Could you check a few things on this model? Use its own coordinates, in mm. A direction names the side the tool comes from. Give positions to 0.01 mm unless a question says otherwise; leave off trailing zeros. Write each loop counter-clockwise with the first axis right and the second up, starting at its lowest first coordinate (ties: lowest second). Pieces come first, ordered by that corner, then holes. Notation, with made-up numbers: (40, 9) - (96, 9) arc R27 ccw to (96, 35) - close; hole circle Ø6 at (75, 41). An arc over 180 degrees is marked (long way). Use one line per item in the form item = value.
Autodesk Inventor part; units mm, degrees
ref_plane "YZ Plane" through (0, 0, 0) normal (1, 0, 0) x (0, 1, 0)
ref_plane "XZ Plane" through (0, 0, 0) normal (0, 1, 0) x (-1, 0, 0)
ref_plane "XY Plane" through (0, 0, 0) normal (0, 0, 1) x (1, 0, 0)
sketch "Sketch1" plane through (0, 0, 0) normal (0, 1, 0) x (-1, 0, 0)
  line L0 (0, 0) -> (22.5, 0)
  line L1 (22.5, 0) -> (22.5, -21)
  line L2 (22.5, -21) -> (0, -21)
  line L3 (0, -21) -> (0, 0)
  circle A0 centre (3, -3) radius 1.5
  circle A1 centre (3, -18) radius 1.5
  line L4 (22.5, -10.5) -> (0, -10.5)
  dimension "d0" = 21
  dimension "d1" = 22.5
  dimension "d2" = 3
  dimension "d5" = 3
  dimension "d8" = 3
  dimension "d25" = 15
  dimension "d26" = 3
extrude "Extrusion1" add sketch "Sketch1" along normal blind 1.5
sketch "Sketch2" plane through (0, 1.5, 0) normal (0, 1, 0) x (1, 0, 0)
  line L0 (-3, 7) -> (-1, 7)
  line L1 (-1, 7) -> (-1, 14)
  line L2 (-1, 14) -> (-3, 14)
  line L3 (-3, 14) -> (-3, 7)
  line L4 (-16.5, 8.25) -> (-16.5, 12.75)
  circle A0 centre (-16.5, 10.5) radius 2.25
  line L5 (-22.5, 21) -> (-22.5, 0)
  line L6 (-22.5, 10.5) -> (0, 10.5)
  line L7 (0, 0) -> (0, 21)
  dimension "d11" = 4.5
  dimension "d12" = 7
  dimension "d13" = 2
  dimension "d14" = 1
  dimension "d15" = 6
extrude "Extrusion2" add sketch "Sketch2" along normal blind 4.5 contours L3 L6 L1 L0 | A0 L4 L6 | L6 L4 A0 | L3 L2 L1 L6 picked at (-15.2379, 9.707) picked at (-15.707, 11.7621)
sketch "Sketch3" plane through (-1, 1.5, -7) normal (1, 0, 0) x (0, 0, -1)
  line L0 (0.5, 3.5) -> (6.5, 3.5)
  line L1 (6.5, 3.5) -> (6.5, 4.5)
  line L2 (6.5, 4.5) -> (0.5, 4.5)
  line L3 (0.5, 4.5) -> (0.5, 3.5)
  line L4 (-7, 0) -> (14, 0)
  line L5 (0, 4.5) -> (7, 4.5)
  line L6 (0, 0) -> (0, 4.5)
  line L7 (7, 0) -> (7, 4.5)
  point P0 (-7, -1.5)
  point P1 (0.5, 4)
  dimension "d18" = 6
  dimension "d19" = 1
  dimension "d21" = 0.5
  dimension "d22" = 0.5
extrude "Extrusion3" add sketch "Sketch3" along normal blind 8 contours L3 L2 L1 L0
properties part number "DS18B20"
1. Imagine slicing it at B-B, the plane y = 4.2. List the corners of the cut face in (x, z) for me.
Response values:
outline = (-16.5, -12.75) arc R2.25 ccw to (-16.5, -8.25) - close; (-3, -14) - (-1, -14) - (-1, -7) - (-3, -7) - close
2. For pin 1 (0.6 mm diameter, centred on x = -2, y = 5, fed in from -Z); pin 2 (1.8 mm diameter, centred on x = 3.5, z = -10, fed in from -Y); pin 3 (1 mm diameter, centred on x = -9, z = -17.5, fed in from +Y); pin 4 (5 mm diameter, centred on x = -1.5, z = -6, fed in from -Y), each with a flat end and sliding along its axis, tell me the tip position at first contact or that it passes through.
Response values:
pin_1 = -14
pin_2 = 5
pin_3 = 1.5
pin_4 = 0
3. If I drill on line 1 (Z direction, x = -3, y = 0.65); line 2 (Y direction, x = -0.5, z = -8.5); line 3 (X direction, y = 5.3, z = -13.75), over which ranges is the centre line in solid material (lowest first)? Write a range as from..to.
Response values:
line_1 = -21..-19.5, -16.5..-4.5, -1.5..0
line_2 = 0..1.5, 5..6
line_3 = -3..-1
4. Which directions (+Z, -Z, +X, -X, +Y, -Y) give clear straight access to the entire face, cutting with the end or side of a thin tool? Please do faces 1 (the face through (-14.25, 3.72, -10.55)), 2 (the face through (-16.5, 4, -10)), 3 (the face through (-2, 4, -7)).
Response values:
face_1 = +Y
face_2 = +Z, -Z, -X, +Y
face_3 = +Z, +X, -X, +Y
5. Imagine slicing it at D-D, the plane z = -5.75. List the corners of the cut face in (x, y) for me, and give its area (4 significant figures).
Response values:
outline = (-22.5, 0) - (0, 0) - (0, 1.5) - (-22.5, 1.5) - close
area = 33.75 mm²
6. Imagine slicing it at C-C, the plane z = -10.5. List the corners of the cut face in (x, y) for me, and give its area (3 significant figures).
Response values:
outline = (-22.5, 0) - (0, 0) - (0, 1.5) - (-1, 1.5) - (-1, 5) - (7, 5) - (7, 6) - (-3, 6) - (-3, 1.5) - (-14.25, 1.5) - (-14.25, 6) - (-16.5, 6) - (-16.5, 1.5) - (-22.5, 1.5) - close
area = 60.9 mm²
7. If we mould it in two halves opening along X, with no side actions, what happens to faces 4 (the face through (0, 1, -11)), 5 (the face through (-2.805, 0.74, -19.487)), 6 (the face through (-11, 1, -21))? For each: pulls with the +X half, pulls with the -X half, needs draft (parallel to the pull), parting line crosses it, or undercut.
Response values:
face_4 = pulls with the +X half
face_5 = undercut
face_6 = needs draft
8. Imagine slicing it at A-A, the plane z = -18. List the corners of the cut face in (x, y) for me.
Response values:
outline = (-22.5, 0) - (-4.5, 0) - (-4.5, 1.5) - (-22.5, 1.5) - close; (-1.5, 0) - (0, 0) - (0, 1.5) - (-1.5, 1.5) - close
